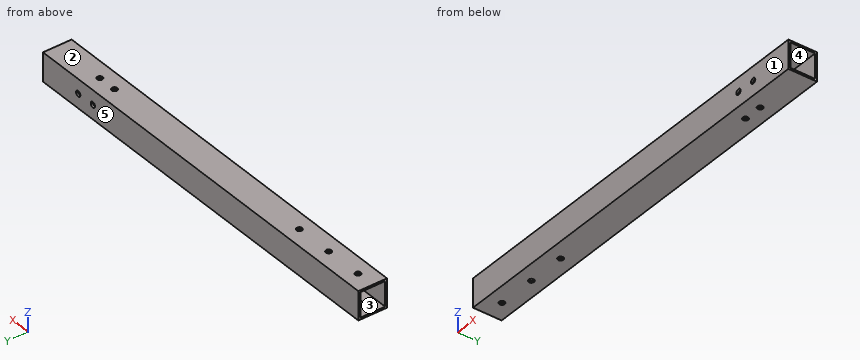
from build123d import *

# Parameters (mm, degrees)
SKETCH_1_W          = 15
SKETCH_1_H          = 15
SKETCH_1_W_2        = 13
SKETCH_1_H_2        = 13
EXTRUDE_1_DEPTH     = 215
SKETCH_2_R          = 1.45
CUT_EXTRUDE_1_DEPTH = 216.653077882
SKETCH_3_R          = 1.45
CUT_EXTRUDE_2_DEPTH = 216.653077882


with BuildPart() as part:
    # 草图1 → 凸台-拉伸1 (new body)
    with BuildSketch(Plane(origin=(0, 0, 0), x_dir=(0, 0, -1), z_dir=(1, 0, 0))):
        Rectangle(SKETCH_1_W, SKETCH_1_H)
        Rectangle(SKETCH_1_W_2, SKETCH_1_H_2, mode=Mode.SUBTRACT)
    extrude(amount=EXTRUDE_1_DEPTH)

    # 草图2 → 切除-拉伸1 (cut, through all)
    with BuildSketch(Plane.XY.offset(7.5)):
        with Locations((50, 0)):
            Circle(SKETCH_2_R)
        with Locations((30, 0)):
            Circle(SKETCH_2_R)
        with Locations((10, 0)):
            Circle(SKETCH_2_R)
        with Locations((186, 0)):
            Circle(SKETCH_2_R)
        with Locations((176, 0)):
            Circle(SKETCH_2_R)
    extrude(amount=-CUT_EXTRUDE_1_DEPTH, mode=Mode.SUBTRACT)

    # 草图3 → 切除-拉伸2 (cut, through all)
    with BuildSketch(Plane(origin=(0, 7.5, 0), x_dir=(1, 0, 0), z_dir=(0, 1, 0))):
        with Locations(Location((191, 0, 0), (0, 0, 270))):
            Circle(SKETCH_3_R)
        with Locations(Location((181, 0, 0), (0, 0, 270))):
            Circle(SKETCH_3_R)
    extrude(amount=-CUT_EXTRUDE_2_DEPTH, mode=Mode.SUBTRACT)


solid = part.part
Geometry check sheet. Reference: the model listing, model coordinates, mm. Face numbers are marked on the shaded views. A direction names the side the tool comes from. Give positions to 0.01 mm unless a question says otherwise; leave off trailing zeros. Loops run counter-clockwise (first coordinate to the right, second up) from the corner with the lowest first, then second, coordinate; pieces in that order, holes last. Notation, with made-up numbers: M -14,75.25 L 42,75.25 A13 ccw 42,85.25 Z; hole C -38.75,-39.5 d11. An arc over 180 degrees is marked long. Write each question's results on one line, items separated by ' | '.
1) Thickness scan on line 1 (Y direction, x = 76.5, z = -5.25); line 2 (X direction, y = -6.9, z = 0). Record the ranges inside material, lowest first.
Answers follow:
line 1: -7.5 to -6.5, 6.5 to 7.5 | line 2: 0 to 179.55, 182.45 to 189.55, 192.45 to 215
2) Release check for a two-part mould opening along Z. For the marked faces 1, 2 and 3 record: +Z half, -Z half, draft (parallel to the pull), parting line (faces both ways), or undercut.
Answers follow:
face 1: draft | face 2: +Z half | face 3: undercut
3) Section check A-A, the plane x = 195. Record the boundary of the cut face in (y, z).
Answers follow:
outline: M -7.5,-7.5 L 7.5,-7.5 L 7.5,7.5 L -7.5,7.5 Z; hole M -6.5,-6.5 L 6.5,-6.5 L 6.5,6.5 L -6.5,6.5 Z
4) Tool access check on the marked faces 4 and 5. Record the directions out of +Z, -Z, +X, -X, +Y, -Y that give a thin tool (end or side, any length) a straight path to the whole face; none if there is none.
Answers follow:
face 4: +X, -X | face 5: +Z, -Z, +X, -X, +Y
